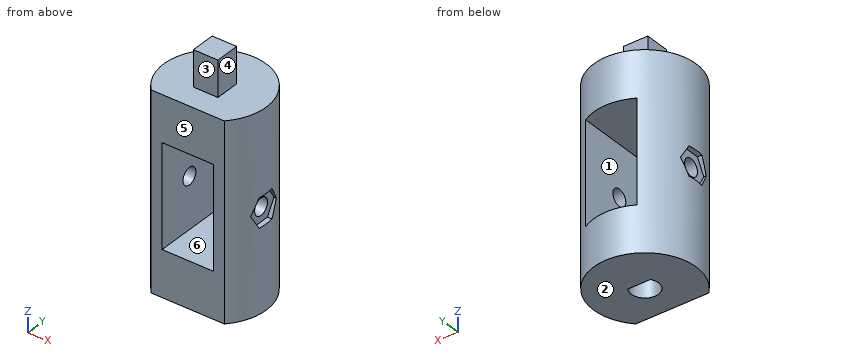
from build123d import *

# Parameters (mm, degrees)
SKIZZE1_R                            = 10
AUFSATZ_LINEAR_AUSTRAGEN1_DEPTH      = 38
SKIZZE2_W                            = 4.8
SKIZZE2_H                            = 4.8
AUFSATZ_LINEAR_AUSTRAGEN2_DEPTH      = 7
SCHNITT_LINEAR_AUSTRAGEN1_DEPTH      = 7
SKIZZE4_W                            = 20
SKIZZE4_H                            = 7
SCHNITT_LINEAR_AUSTRAGEN3_DEPTH      = 38
SCHNITT_LINEAR_AUSTRAGEN4_REACH      = 19
SKIZZE5_W                            = 10
SKIZZE5_H                            = 20
SKIZZE6_R                            = 1.65
SCHNITT_LINEAR_AUSTRAGEN5_DEPTH      = 16
SCHNITT_LINEAR_AUSTRAGEN5_DEPTH_BACK = 6
SCHNITT_LINEAR_AUSTRAGEN6_REACH      = 11
SCHNITT_LINEAR_START                 = -4
SCHNITT_LINEAR_AUSTRAGEN7_REACH      = 31
SCHNITT_LINEAR_START_2               = 14


with BuildPart() as part:
    # Skizze1 → Aufsatz-Linear austragen1 (new body)
    with BuildSketch(Plane.XY):
        Circle(SKIZZE1_R)
    extrude(amount=AUFSATZ_LINEAR_AUSTRAGEN1_DEPTH)

    # Skizze2 → Aufsatz-Linear austragen2 (add)
    with BuildSketch(Plane.XY.offset(38)):
        Rectangle(SKIZZE2_W, SKIZZE2_H)
    extrude(amount=AUFSATZ_LINEAR_AUSTRAGEN2_DEPTH)

    # Skizze3 → Schnitt-Linear austragen1 (cut)
    with BuildSketch(Plane(origin=(0, 0, 0), x_dir=(-1, 0, 0), z_dir=(0, 0, -1))):
        with BuildLine():
            Line((2.184605227, 1.5), (-2.184605227, 1.5))
            ThreePointArc((-2.184605227, 1.5), (-0.785269427, -2.530978452), (2.65, 0))
            ThreePointArc((2.65, 0), (2.530978452, 0.785269427), (2.184605227, 1.5))
        make_face()
    extrude(amount=-SCHNITT_LINEAR_AUSTRAGEN1_DEPTH, mode=Mode.SUBTRACT)

    # Skizze4 → Schnitt-Linear austragen3 (cut)
    with BuildSketch(Plane(origin=(0, 0, 0), x_dir=(-1, 0, 0), z_dir=(0, 0, -1))):
        with Locations((0, -10.5)):
            Rectangle(SKIZZE4_W, SKIZZE4_H)
    extrude(amount=-SCHNITT_LINEAR_AUSTRAGEN3_DEPTH, mode=Mode.SUBTRACT)

    # Skizze5 → Schnitt-Linear austragen4 (cut, up to next)
    with BuildSketch(Plane.XZ.offset(7), mode=Mode.PRIVATE) as schnitt_linear_austragen4_sk1:
        with Locations((0, 19)):
            Rectangle(SKIZZE5_W, SKIZZE5_H)
    schnitt_linear_austragen4_tool1 = extrude(schnitt_linear_austragen4_sk1.sketch, amount=-SCHNITT_LINEAR_AUSTRAGEN4_REACH, mode=Mode.PRIVATE) & part.part
    add(schnitt_linear_austragen4_tool1.solids().sort_by_distance((0, -7, 19))[0], mode=Mode.SUBTRACT)

    # Skizze6 → Schnitt-Linear austragen5 (cut, two sides)
    with BuildSketch(Plane.ZY.offset(-5)) as schnitt_linear_austragen5_sk:
        with Locations((19, 0)):
            Circle(SKIZZE6_R)
    extrude(amount=SCHNITT_LINEAR_AUSTRAGEN5_DEPTH, mode=Mode.SUBTRACT)
    extrude(schnitt_linear_austragen5_sk.sketch, amount=-SCHNITT_LINEAR_AUSTRAGEN5_DEPTH_BACK, mode=Mode.SUBTRACT)

    # Skizze7 → Schnitt-Linear austragen6 (cut, up to next)
    with BuildSketch(Plane.ZY.offset(-5).offset(SCHNITT_LINEAR_START), mode=Mode.PRIVATE) as schnitt_linear_austragen6_sk1:
        Polygon((19, -3.290896534), (21.85, -1.645448267), (21.85, 1.645448267), (19, 3.290896534), (16.15, 1.645448267), (16.15, -1.645448267), align=None)
    schnitt_linear_austragen6_tool1 = extrude(schnitt_linear_austragen6_sk1.sketch, amount=-SCHNITT_LINEAR_AUSTRAGEN6_REACH, mode=Mode.PRIVATE) & part.part
    add(schnitt_linear_austragen6_tool1.solids().sort_by_distance((9, 0, 19))[0], mode=Mode.SUBTRACT)

    # Skizze7<2> → Schnitt-Linear austragen7 (cut, up to next)
    with BuildSketch(Plane.ZY.offset(-5).offset(SCHNITT_LINEAR_START_2), mode=Mode.PRIVATE) as schnitt_linear_austragen7_sk1:
        Polygon((19, -3.290896534), (21.85, -1.645448267), (21.85, 1.645448267), (19, 3.290896534), (16.15, 1.645448267), (16.15, -1.645448267), align=None)
    schnitt_linear_austragen7_tool1 = extrude(schnitt_linear_austragen7_sk1.sketch, amount=SCHNITT_LINEAR_AUSTRAGEN7_REACH, mode=Mode.PRIVATE) & part.part
    add(schnitt_linear_austragen7_tool1.solids().sort_by_distance((-9, 0, 19))[0], mode=Mode.SUBTRACT)


solid = part.part
For this review, take the finished solid that the model builds, in its own axes (mm). Face numbers are marked on the shaded views. A direction names the side the tool comes from. Give positions to 0.01 mm unless a question says otherwise; leave off trailing zeros. Loops run counter-clockwise (first coordinate to the right, second up) from the corner with the lowest first, then second, coordinate; pieces in that order, holes last. Notation, with made-up numbers: M 21.25,-32.75 L 25.25,-32.75 A19 cw 25.25,-26.75 Z; hole C 16,69.5 d3. An arc over 180 degrees is marked long. Put each result on its own line as item: value. Start each with the question number.
(1) Add section D-D, the plane z = 6.5. Write out the cut boundary in (x, y), then the cut area to 3 significant figures.
(2) For pin 1 (8 mm diameter, centred on x = 6.5, y = 1, fed in from -Z); pin 2 (1.2 mm diameter, centred on x = -1, y = -0.5, fed in from -Z); pin 3 (4.5 mm diameter, centred on y = 4.5, z = 20, fed in from +X); pin 4 (4.5 mm diameter, centred on y = 1.5, z = 20, fed in from -X), all flat-tipped, find the tip position at first contact; note any pin that passes through.
(3) The part is to be moulded in two halves that separate along X. For the marked faces 4, 5 and 6, say which applies: +X half, -X half, draft (parallel to the pull), parting line (faces both ways), or undercut.
(4) Add section C-C, the plane z = 12. Write out the cut boundary in (x, y).
(5) Add section B-B, the plane x = -1.75. Write out the cut boundary in (y, z).
(6) Machinability: for the marked faces 1, 2 and 3, which of the approach directions +Z, -Z, +X, -X, +Y, -Y give a long, thin tool a straight path to every point of the face, cutting with its end or side? Answer none if there is none.
(7) Add section A-A, the plane z = 19.5. Write out the cut boundary in (x, y).
(8) Wall thickness on L1, parallel to Z at x = 3.75, y = 8; L2, parallel to Z at x = -6.6, y = 0; L3, parallel to Y at x = 0, z = 3: over which ranges is each line inside the solid? List them lowest first.
Result:
1. outline: M -7.14,-7 L 7.14,-7 A10 ccw long Z; hole M -2.18,1.5 A2.65 ccw long 2.18,1.5 Z
1. area: 266 mm^2
2. pin 1: stops at z = 0
2. pin 2: stops at z = 7
2. pin 3: stops at x = 9.72
2. pin 4: stops at x = -10
3. face 4: +X half
3. face 5: draft
3. face 6: undercut
4. outline: M -7.14,-7 L -5,-7 L -5,8.66 A10 ccw Z; M 5,-7 L 7.14,-7 A10 ccw 5,8.66 Z
5. outline: M -7,0 L -1.99,0 L -1.99,7 L 1.5,7 L 1.5,0 L 9.85,0 L 9.85,9 L -7,9 Z; M -7,29 L 9.85,29 L 9.85,38 L 2.4,38 L 2.4,45 L -2.4,45 L -2.4,38 L -7,38 Z
6. face 1: +Y, -Y
6. face 2: -Z, +X, -X, +Y, -Y
6. face 3: +Z, +X, -X, -Y
7. outline: M -9.54,-3 A10 ccw -7.14,-7 L -5,-7 L -5,-1.57 L -9,-1.57 L -9,-3 Z; M -9.54,3 L -9,3 L -9,1.57 L -5,1.57 L -5,8.66 A10 ccw Z; M 5,-7 L 7.14,-7 A10 ccw 9.54,-3 L 9,-3 L 9,-1.57 L 5,-1.57 Z; M 5,1.57 L 9,1.57 L 9,3 L 9.54,3 A10 ccw 5,8.66 Z
8. L1: z = 0 to 9, 29 to 38
8. L2: z = 0 to 17.35, 20.65 to 38
8. L3: y = -7 to -2.65, 1.5 to 10
